```python
from build123d import *

# Parameters (mm, degrees)
SKETCH1_W           = 30
SKETCH1_H           = 25
BOSS_EXTRUDE1_DEPTH = 20
SKETCH2_W           = 20
SKETCH2_H           = 25
CUT_EXTRUDE1_DEPTH  = 10
CUT_EXTRUDE2_DEPTH  = 20
CUT_EXTRUDE3_DEPTH  = 40
SKETCH5_W           = 10
SKETCH5_H           = 10.001690502
CUT_EXTRUDE4_DEPTH  = 20


with BuildPart() as part:
    # Sketch1 → Boss-Extrude1 (new body)
    with BuildSketch(Plane.XY):
        with Locations((15, 12.5)):
            Rectangle(SKETCH1_W, SKETCH1_H)
    extrude(amount=BOSS_EXTRUDE1_DEPTH)

    # Sketch2 → Cut-Extrude1 (cut)
    with BuildSketch(Plane.XY.offset(20)):
        with Locations((10, 12.5)):
            Rectangle(SKETCH2_W, SKETCH2_H)
    extrude(amount=-CUT_EXTRUDE1_DEPTH, mode=Mode.SUBTRACT)

    # Sketch3 → Cut-Extrude2 (cut)
    with BuildSketch(Plane.ZY.offset(-20)):
        Polygon((15, 25), (20, 15), (20, 25), align=None)
    extrude(amount=-CUT_EXTRUDE2_DEPTH, mode=Mode.SUBTRACT)

    # Sketch4 → Cut-Extrude3 (cut)
    with BuildSketch(Plane(origin=(0, 25, 0), x_dir=(1, 0, 0), z_dir=(0, 1, 0))):
        Polygon((0, -10), (10, -10), (0, 0), align=None)
    extrude(amount=-CUT_EXTRUDE3_DEPTH, mode=Mode.SUBTRACT)

    # Sketch5 → Cut-Extrude4 (cut)
    with BuildSketch(Plane.XY.offset(10)):
        with Locations((5, 19.999154749)):
            Rectangle(SKETCH5_W, SKETCH5_H)
    extrude(amount=-CUT_EXTRUDE4_DEPTH, mode=Mode.SUBTRACT)


solid = part.part
```
Part model, mm, in its own coordinate system. A direction names the side the tool comes from. Round coordinates to 2 decimals unless told otherwise and drop trailing zeros. Order: outer loops, then holes, each group sorted by start corner. A loop starts at its lowest first (then second) coordinate and runs counter-clockwise, first axis right, second up. Notation, with made-up numbers: M 60,-33 L 69,-33 A32 cw 69,-2 Z; hole C 2,-2.5 d6. An arc over 180 degrees is marked long. Put each result on its own line as item: value. Start each with the question number.
1. Slice it at B-B on z = 4.25. List the corners of the cut face in (x, y).
2. Tool access for faces 1 (the face through (30, 12, 10)), 2 (the face through (10, 20, 5)), 3 (the face through (20, 12, 15)): list every direction of +Z, -Z, +X, -X, +Y, -Y with a clear straight run to the whole face (end or side of a thin tool).
3. Drill centre lines: probe 1 along Y at (x, z) = (5.75, 1.25); probe 2 along Z at (x, y) = (18.5, 20.25); probe 3 along X at (y, z) = (20.5, 14.5). Where is each one in solid material? Low to high. Write a range as [from, to].
4. Drop flat-ended pins along their axis: pin 1 (6 mm diameter, centred on x = 6, y = 9.5, fed in from -Z); pin 2 (5 mm diameter, centred on y = 22, z = 3.5, fed in from -X); pin 3 (8 mm diameter, centred on y = 18, z = 17, fed in from -X). Give the stop position or say it passes through.
5. Slice it at A-A on y = 11. List the corners of the cut face in (x, z), then the cut area to 3 significant figures.
6. Slice it at D-D on z = 15.75. List the corners of the cut face in (x, y), then the cut area to 3 significant figures.
7. Slice it at C-C on x = 21.75. List the corners of the cut face in (y, z).
Findings:
1. outline: M 4.25,0 L 30,0 L 30,25 L 10,25 L 10,15 L 4.25,15 Z
2. face 1: +Z, -Z, +X, +Y, -Y
2. face 2: +Z, -Z, -X, +Y
2. face 3: +Z, -X, +Y, -Y
3. probe 1: [0, 15]
3. probe 2: [0, 10]
3. probe 3: [20, 30]
4. pin 1: z = 0
4. pin 2: x = 10
4. pin 3: x = 20
5. outline: M 0,0 L 30,0 L 30,20 L 20,20 L 20,10 L 10,10 Z
5. area: 350 mm2
6. outline: M 20,0 L 30,0 L 30,23.5 L 20,23.5 Z
6. area: 235 mm2
7. outline: M 0,0 L 25,0 L 25,15 L 15,20 L 0,20 Z
